```python
from build123d import *

# Parameters (mm, degrees)
F0_R     = 21.5
F1_DEPTH = 20
F2_R     = 19.0313090647
F3_DEPTH = 0.5
F4_R     = 19.0313090647
F5_DEPTH = 40


# Not quite as in the source:
# - a fillet or chamfer that OpenCascade refuses, or shapes differently, is made with other operations: its cross-section is extruded or revolved along the edge and cut away or added


with BuildPart() as f1:
    # F0 (on Top) → F1 (new body)
    with BuildSketch(Plane.XY):
        Circle(F0_R)
    extrude(amount=F1_DEPTH)

    # F2 (on face) → F3 (join)
    with BuildSketch(Plane(origin=(0, 0, 0), x_dir=(1, 0, 0), z_dir=(0, 0, -1))):
        Circle(F2_R)
    extrude(amount=F3_DEPTH)

    # F4 (on face) → F5 (join)
    with BuildSketch(Plane(origin=(0, 0, -0.5), x_dir=(1, 0, 0), z_dir=(0, 0, -1))):
        Circle(F4_R)
    extrude(amount=F5_DEPTH)

    # F6: chamfer of 2.5 x 30 on 1 edges, made by hand

    # F6_s1 → F6_t2 (revolve, cut)
    with BuildSketch(Plane.XZ):
        Polygon((19.0313090647, -10.5), (16.5313090647, -40.5), (19.0313090647, -40.5), align=None)
    revolve(axis=Axis((0, 0, -40.5), (0, 0, -1)), mode=Mode.SUBTRACT)

    # F7: fillet of radius 5 on 2 edges, made by hand

    # F7_s1 → F7_t2 (revolve, cut)
    with BuildSketch(Plane.XZ):
        with BuildLine():
            ThreePointArc((16.9133734481, -35.9152273993), (15.3161921018, -39.1794114337), (11.9306446569, -40.5))
            Line((11.9306446569, -40.5), (16.5313090647, -40.5))
            Line((16.5313090647, -40.5), (16.9133734481, -35.9152273993))
        make_face()
    revolve(axis=Axis((0, 0, -40.5), (0, 0, -1)), mode=Mode.SUBTRACT)

    # F7_s3 → F7_t4 (revolve, cut)
    with BuildSketch(Plane.XZ):
        with BuildLine():
            ThreePointArc((19.0313090647, -10.2920271064), (19.0269893965, -10.4998203255), (19.0140378559, -10.7072545056))
            Line((19.0140378559, -10.7072545056), (19.0313090647, -10.5))
            Line((19.0313090647, -10.5), (19.0313090647, -10.2920271064))
        make_face()
    revolve(axis=Axis((0, 0, -10.5), (0, 0, -1)), mode=Mode.SUBTRACT)


solid = f1.part
```
Check sheet for the modelled part. Datum: model origin and axes. Units: mm. A direction names the side the tool comes from. Round coordinates to 2 decimals unless told otherwise and drop trailing zeros. Loops run counter-clockwise (first coordinate to the right, second up) from the corner with the lowest first, then second, coordinate; pieces in that order, holes last. Notation, with made-up numbers: (40.5, 65) - (65.5, 65) arc R21 cw to (65.5, 90) - close; hole circle Ø5 at (-36.5, 22). An arc over 180 degrees is marked (long way). Write item = value, one per line. Start each with the question number.
Q1. Section check C-C (z = -22). Record the boundary of the cut face in (x, y), plus the area to 3 significant figures.
Q2. Section check A-A (x = 0). Record the boundary of the cut face in (y, z).
Q3. Access from +Z, -Z, +X, -X, +Y, -Y to the whole of each face (thin tool, end or side, straight path). Record for faces 1 (the face through (0, 0, 20)), 2 (the face through (-4.126, 18.579, -5.074)).
Q4. Section check D-D (z = -35). Record the boundary of the cut face in (x, y), plus the area to 3 significant figures.
Q5. Thickness scan on L1, parallel to Z at x = -14.5, y = 13; L2, parallel to Y at x = 0, z = 15.5; L3, parallel to Y at x = -12.5, z = 8.5. Record the ranges inside material, lowest first.
Q6. Depth check by flat-ended pin: P1, Ø5, axis at x = -14, z = -34, coming from the -Y side; P2, Ø4, axis at x = -13.5, z = -15, coming from the -Y side; P3, Ø6, axis at x = -6, z = -30, coming from the +Y side. Enter the tip coordinate at first touch or a pass-through.
Derived:
q1.outline = circle Ø36.15 at (0, 0)
q1.area = 1,030 mm^2
q2.outline = (-21.5, 0) - (-19.03, 0) - (-19.03, -10.29) arc R5 ccw to (-19.01, -10.71) - (-16.91, -35.92) arc R5 ccw to (-11.93, -40.5) - (11.93, -40.5) arc R5 ccw to (16.91, -35.92) - (19.01, -10.71) arc R5 ccw to (19.03, -10.29) - (19.03, 0) - (21.5, 0) - (21.5, 20) - (-21.5, 20) - close
q3.face_1 = +Z, +X, -X, +Y, -Y
q3.face_2 = -Z
q4.outline = circle Ø33.98 at (0, 0)
q4.area = 907 mm^2
q5.L1 = 0 to 20
q5.L2 = -21.5 to 21.5
q5.L3 = -17.49 to 17.49
q6.P1 = -12.64
q6.P2 = -14.7
q6.P3 = 17.2
